Geometry check sheet. Reference: the model listing, model coordinates, mm. Give positions to 0.01 mm unless a question says otherwise; leave off trailing zeros. Order: outer loops, then holes, each group sorted by start corner. A loop starts at its lowest first (then second) coordinate and runs counter-clockwise, first axis right, second up. Notation, with made-up numbers: M 40.5,79 L 51.5,79 A17 ccw 51.5,100 Z; hole C -20.5,55 d10. An arc over 180 degrees is marked long. Answer as CSV lines item,"result". Start each with the question number.
Q1. Mould release check, pull along Z, two halves, no side actions. Record for faces 1 (the flat face through (2, 43, 0)), 2 (the cylindrical face through (1.61, 31.573, -35.166)), 3 (the flat face through (2, 0, -34)): +Z half, -Z half, draft (parallel to the pull), parting line (faces both ways), or undercut.
Q2. Go/stop test with a flat-tipped pin: pin 1 (8 mm diameter, centred on y = 21.19, z = -27.34, fed in from -X). Record where the tip stops, or that it passes through.
Q3. Section check B-B, the plane z = -28.5. Record the boundary of the cut face in (x, y) (3 decimals).
Q4. Section check A-A, the plane x = 0.95. Count the separate pieces of the cut face and the enclosed holes in it, then the cut area to 3 significant figures.
Q5. Thickness scan on line 1 (Y direction, x = 0.65, z = -37.5); line 2 (Y direction, x = 2.15, z = -14.5); line 3 (Z direction, x = 0.3, y = 27). Record the ranges inside material, lowest first.
```python
from build123d import *

# Parameters (mm, degrees)
SKETCH1_W                           = 69.85
SKETCH1_H                           = 86.36
BOSS_EXTRUDE1_DEPTH                 = 3.175
F_1_2_CLEARANCE_HOLE1_D             = 13.09624
F_1_2_CLEARANCE_HOLE1_DEPTH         = 25.4
F_1_2_CLEARANCE_HOLE1_TIP           = 3.934507437
M3_CLEARANCE_HOLE1_D                = 3.2
M3_CLEARANCE_HOLE1_DEPTH            = 25.4
M3_CLEARANCE_HOLE1_TIP              = 0.96137699
F_2_0MM_CLEARANCE_DOWEL_HOLE1_D     = 2
F_2_0MM_CLEARANCE_DOWEL_HOLE1_DEPTH = 25.4
F_2_0MM_CLEARANCE_DOWEL_HOLE1_TIP   = 0.600860619


with BuildPart() as part:
    # Sketch1 → Boss-Extrude1 (new body)
    with BuildSketch(Plane(origin=(0, 0, 0), x_dir=(0, 0, -1), z_dir=(1, 0, 0))):
        with Locations((34.925, 43.18)):
            Rectangle(SKETCH1_W, SKETCH1_H)
    extrude(amount=BOSS_EXTRUDE1_DEPTH)

    # 1/2 Clearance Hole1
    with Locations(Plane(origin=(3.175, 0, 0), x_dir=(0, 0, -1), z_dir=(1, 0, 0))):
        with Locations((27.33778886, 21.18693756)):
            Hole(F_1_2_CLEARANCE_HOLE1_D / 2, depth=F_1_2_CLEARANCE_HOLE1_DEPTH)
            with Locations((0, 0, -(F_1_2_CLEARANCE_HOLE1_DEPTH + F_1_2_CLEARANCE_HOLE1_TIP / 2))):  # 118° drill point
                Cone(0, F_1_2_CLEARANCE_HOLE1_D / 2, F_1_2_CLEARANCE_HOLE1_TIP, mode=Mode.SUBTRACT)

    # M3 Clearance Hole1
    with Locations(Plane.ZY):
        with Locations((-40.03778886, 21.18693756), (-33.68778886, 32.185460188), (-20.98778886, 32.185460188), (-14.63778886, 21.18693756), (-20.98778886, 10.188414932), (-33.68778886, 10.188414932), (-27.33778886, 21.18693756)):
            Hole(M3_CLEARANCE_HOLE1_D / 2, depth=M3_CLEARANCE_HOLE1_DEPTH)
            with Locations((0, 0, -(M3_CLEARANCE_HOLE1_DEPTH + M3_CLEARANCE_HOLE1_TIP / 2))):  # 118° drill point
                Cone(0, M3_CLEARANCE_HOLE1_D / 2, M3_CLEARANCE_HOLE1_TIP, mode=Mode.SUBTRACT)

    # Ø2.0mm Clearance Dowel Hole1
    with Locations(Plane(origin=(3.175, 0, 0), x_dir=(0, 0, -1), z_dir=(1, 0, 0))):
        with Locations((37.59058776, 24.95127344)):
            Hole(F_2_0MM_CLEARANCE_DOWEL_HOLE1_D / 2, depth=F_2_0MM_CLEARANCE_DOWEL_HOLE1_DEPTH)
            with Locations((0, 0, -(F_2_0MM_CLEARANCE_DOWEL_HOLE1_DEPTH + F_2_0MM_CLEARANCE_DOWEL_HOLE1_TIP / 2))):  # 118° drill point
                Cone(0, F_2_0MM_CLEARANCE_DOWEL_HOLE1_D / 2, F_2_0MM_CLEARANCE_DOWEL_HOLE1_TIP, mode=Mode.SUBTRACT)


solid = part.part
```
Answer block:
1,face 1,"+Z half"
1,face 2,"undercut"
1,face 3,"draft"
2,pin 1,"passes through"
3,outline,"M 0,0 L 3.175,0 L 3.175,14.743 L 0,14.743 Z; M 0,27.631 L 3.175,27.631 L 3.175,86.36 L 0,86.36 Z"
4,separate pieces,"1"
4,enclosed holes,"8"
4,area,"5,850 mm2"
5,line 1,"y = 0 to 23.96, 25.95 to 86.36"
5,line 2,"y = 0 to 19.59, 22.78 to 86.36"
5,line 3,"z = -69.85 to -30.35, -24.32 to 0"
